from build123d import *

# Parameters (mm, degrees)
BOSS_EXTRUDE1_DEPTH     = 6.35
CUT_EXTRUDE1_DEPTH      = 119.1487118
CUT_EXTRUDE1_DEPTH_BACK = 119.1487118
SKETCH3_R               = 6.35


with BuildPart() as part:
    # Sketch1 → Boss-Extrude1 (new body)
    with BuildSketch(Plane.XY):
        Polygon((-20, 0), (20, 0), (20, 30), (26.34, 30), (26.34, 50), (20, 50), (20, 80), (26.34, 80), (26.34, 100), (20, 100), (20, 115), (-20, 115), (-20, 100), (-26.34, 100), (-26.34, 80), (-20, 80), (-20, 50), (-26.34, 50), (-26.34, 30), (-20, 30), align=None)
    extrude(amount=BOSS_EXTRUDE1_DEPTH)

    # Sketch3 → Cut-Extrude1 (cut, two sides: drawn at the far end of the back side and taken through both)
    with BuildSketch(Plane.XY.offset(6.35).offset(-CUT_EXTRUDE1_DEPTH_BACK)):
        with Locations((0, 90)):
            Circle(SKETCH3_R)
        with Locations((0, 40)):
            Circle(SKETCH3_R)
    extrude(amount=CUT_EXTRUDE1_DEPTH + CUT_EXTRUDE1_DEPTH_BACK, mode=Mode.SUBTRACT)


solid = part.part
Source: CAD feature listing. Evaluate the final solid. Frame: model axes, mm. A direction names the side the tool comes from. Round coordinates to 2 decimals unless told otherwise and drop trailing zeros. Loops run counter-clockwise (first coordinate to the right, second up) from the corner with the lowest first, then second, coordinate; pieces in that order, holes last. Notation, with made-up numbers: M -23,86 L -9,86 A15 cw -9,114 Z; hole C -2.5,-29 d6. An arc over 180 degrees is marked long. Return JSON: item names as keys, results as strings. Group by question number.
1. Section query D-D on y = 102.5. Output: boundary loops of the cut face in (x, z), and give its area (3 significant figures).
2. Section query C-C on x = 0. Output: boundary loops of the cut face in (y, z), and give its area (3 significant figures).
3. Pin query (flat end, axial travel): pin 1 (1.9 mm diameter, centred on y = 62, z = 4.5, fed in from -X); pin 2 (3 mm diameter, centred on y = 66, z = 2, fed in from +X); pin 3 (3 mm diameter, centred on x = 6, y = 98, fed in from -Z); pin 4 (1.9 mm diameter, centred on x = 22, z = 1.5, fed in from -Y). Return the tip coordinate at first contact, or that it passes through.
4. Reachability of faces 1 (the face through (23, 100, 3)), 2 (the face through (-20, 65, 3)), 3 (the face through (23, 30, 3)), 4 (the face through (23, 50, 3)) from +Z, -Z, +X, -X, +Y, -Y: full face, straight path, thin tool, end or side. Return the list, or none.
5. Material intervals for line 1 along Y through (x, z) = (0, 5.25); line 2 along X through (y, z) = (90, 2.75); line 3 along Y through (x, z) = (-5, 6), sorted ascending. Write a range as from..to.
6. Section query A-A on z = 2. Output: boundary loops of the cut face in (x, y).
7. Section query B-B on y = 40. Output: boundary loops of the cut face in (x, z), and give its area (3 significant figures).
Checks:
{
 "1": {"outline": "M -20,0 L 20,0 L 20,6.35 L -20,6.35 Z", "area": "254 mm²"},
 "2": {"outline": "M 0,0 L 33.65,0 L 33.65,6.35 L 0,6.35 Z; M 46.35,0 L 83.65,0 L 83.65,6.35 L 46.35,6.35 Z; M 96.35,0 L 115,0 L 115,6.35 L 96.35,6.35 Z", "area": "569 mm²"},
 "3": {"pin 1": "stops at x = -20", "pin 2": "stops at x = 20", "pin 3": "stops at z = 0", "pin 4": "stops at y = 30"},
 "4": {"face 1": "+Z, -Z, +X, +Y", "face 2": "+Z, -Z, -X", "face 3": "+Z, -Z, +X, -Y", "face 4": "+Z, -Z, +X"},
 "5": {"line 1": "y = 0..33.65, 46.35..83.65, 96.35..115", "line 2": "x = -26.34..-6.35, 6.35..26.34", "line 3": "y = 0..36.09, 43.91..86.09, 93.91..115"},
 "6": {"outline": "M -26.34,30 L -20,30 L -20,0 L 20,0 L 20,30 L 26.34,30 L 26.34,50 L 20,50 L 20,80 L 26.34,80 L 26.34,100 L 20,100 L 20,115 L -20,115 L -20,100 L -26.34,100 L -26.34,80 L -20,80 L -20,50 L -26.34,50 Z; hole C 0,40 d12.7; hole C 0,90 d12.7"},
 "7": {"outline": "M -26.34,0 L -6.35,0 L -6.35,6.35 L -26.34,6.35 Z; M 6.35,0 L 26.34,0 L 26.34,6.35 L 6.35,6.35 Z", "area": "254 mm²"}
}
